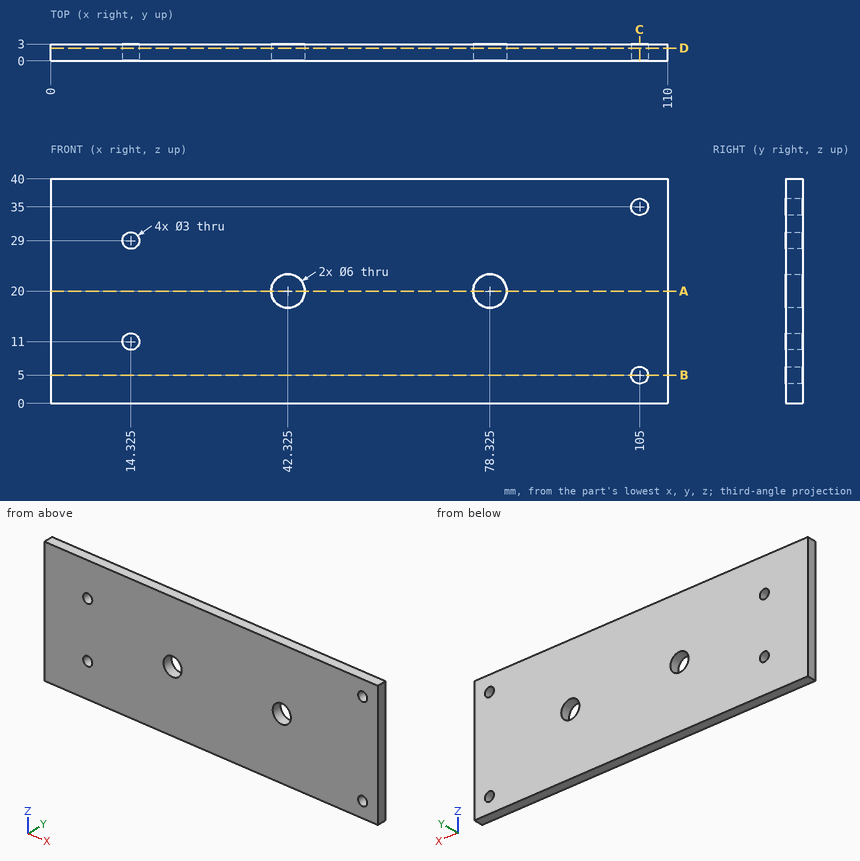
Design review of the part shown in the three views and the two pictorial views. Dimensions are in mm from the part's minimum x, y and z. Round coordinates to 2 decimals unless told otherwise and drop trailing zeros. Write each loop counter-clockwise with the first axis right and the second up, starting at its lowest first coordinate (ties: lowest second). Pieces come first, ordered by that corner, then holes.
Item 1: For probe 1 along X at (y, z) = (2.1, 20) (3 decimals); probe 2 along X at (y, z) = (2.25, 11) (3 decimals); probe 3 along Z at (x, y) = (105, 1.15), list the stretches that pass through material, from the lowest coordinate up.
Item 2: We need section C-C on x = 105. Write out the cut boundary in (y, z), and give its area (3 significant figures).
Item 3: We need section B-B on z = 5. Write out the cut boundary in (x, y), and give its area (3 significant figures).
Item 4: We need section A-A on z = 20. Write out the cut boundary in (x, y) (3 decimals).
Item 5: We need section D-D on y = 2.25. Write out the cut boundary in (x, z) (3 decimals), and give its area (3 significant figures).
Returned:
1. probe 1: x = 0 to 39.325, 45.325 to 75.325, 81.325 to 110
1. probe 2: x = 0 to 12.825, 15.825 to 110
1. probe 3: z = 0 to 3.5, 6.5 to 33.5, 36.5 to 40
2. outline: (0, 0) - (3, 0) - (3, 3.5) - (0, 3.5) - close; (0, 6.5) - (3, 6.5) - (3, 33.5) - (0, 33.5) - close; (0, 36.5) - (3, 36.5) - (3, 40) - (0, 40) - close
2. area: 102 mm2
3. outline: (0, 0) - (103.5, 0) - (103.5, 3) - (0, 3) - close; (106.5, 0) - (110, 0) - (110, 3) - (106.5, 3) - close
3. area: 321 mm2
4. outline: (0, 0) - (39.325, 0) - (39.325, 3) - (0, 3) - close; (45.325, 0) - (75.325, 0) - (75.325, 3) - (45.325, 3) - close; (81.325, 0) - (110, 0) - (110, 3) - (81.325, 3) - close
5. outline: (0, 0) - (110, 0) - (110, 40) - (0, 40) - close; hole circle Ø3 at (14.325, 11); hole circle Ø3 at (14.325, 29); hole circle Ø6 at (42.325, 20); hole circle Ø6 at (78.325, 20); hole circle Ø3 at (105, 5); hole circle Ø3 at (105, 35)
5. area: 4,320 mm2
